```python
from build123d import *
from build123d.topology import SkipClean

# Parameters (mm, degrees)
SKETCH1_R                    = 4
COUPLER_SECTION_DEPTH        = 12.5
SKETCH3_R                    = 5
BEARING_SECTION_DEPTH        = 12
SKETCH4_R                    = 7
BEARING_STOP_DEPTH           = 3
SKETCH5_R                    = 4
SMALL_SEAL_SECTION_DEPTH     = 12.3
SET_SCREW_FLAT_SECTION_DEPTH = 10.5
SKETCH7_R                    = 4
IMPELLER_SECTION_DEPTH       = 22.163925
SKETCH8_R                    = 1.5
CUT_EXTRUDE1_DEPTH           = 8
CUT_EXTRUDE2_DEPTH           = 23
CUT_EXTRUDE2_DEPTH_BACK      = 23
SKETCH9_R                    = 1


with BuildPart() as part:
    # Sketch1 → coupler section (new body)
    with BuildSketch(Plane(origin=(0, 0, 0), x_dir=(1, 0, 0), z_dir=(0, 1, 0))):
        with Locations(Location((0, 0, 0), (0, 0, 270))):
            Circle(SKETCH1_R)
    extrude(amount=COUPLER_SECTION_DEPTH)

    # Sketch3 → bearing section (add)
    with BuildSketch(Plane(origin=(0, 12.5, 0), x_dir=(1, 0, 0), z_dir=(0, 1, 0))):
        with Locations(Location((0, 0, 0), (0, 0, 270))):
            Circle(SKETCH3_R)
    extrude(amount=BEARING_SECTION_DEPTH)

    # Sketch4 → bearing stop (add)
    with BuildSketch(Plane(origin=(0, 24.5, 0), x_dir=(1, 0, 0), z_dir=(0, 1, 0))):
        with Locations(Location((0, 0, 0), (0, 0, 270))):
            Circle(SKETCH4_R)
    extrude(amount=BEARING_STOP_DEPTH)

    # Sketch5 → small seal section (add)
    with BuildSketch(Plane(origin=(0, 27.5, 0), x_dir=(1, 0, 0), z_dir=(0, 1, 0))):
        with Locations(Location((0, 0, 0), (0, 0, 270))):
            Circle(SKETCH5_R)
    extrude(amount=SMALL_SEAL_SECTION_DEPTH)

    # Sketch6 → set screw flat section (cut)
    with BuildSketch(Plane.XZ):
        with BuildLine():
            Line((-2.645751311, 3), (2.645751311, 3))
            ThreePointArc((2.645751311, 3), (0, 4), (-2.645751311, 3))
        make_face()
    extrude(amount=-SET_SCREW_FLAT_SECTION_DEPTH, mode=Mode.SUBTRACT)

    # Sketch7 → impeller section (add)
    with BuildSketch(Plane(origin=(0, 39.8, 0), x_dir=(1, 0, 0), z_dir=(0, 1, 0))):
        with Locations(Location((0, 0, 0), (0, 0, 311.409622109))):
            Circle(SKETCH7_R)
    extrude(amount=IMPELLER_SECTION_DEPTH)

    # Sketch8 → Cut-Extrude1 (cut)
    with BuildSketch(Plane(origin=(0, 61.963925, 0), x_dir=(1, 0, 0), z_dir=(0, 1, 0))):
        with Locations(Location((0, 0, 0), (0, 0, 270))):
            Circle(SKETCH8_R)
    extrude(amount=-CUT_EXTRUDE1_DEPTH, mode=Mode.SUBTRACT)

    # Sketch9 → Cut-Extrude2 (cut, two sides: drawn at the far end of the back side and taken through both)
    with SkipClean():  # the faces are left unmerged after this step: merging them gives an invalid solid
        with BuildSketch(Plane.XY.offset(-CUT_EXTRUDE2_DEPTH_BACK)):
            with Locations(Location((0, 42.963925, 0), (0, 0, 89.999999996))):
                Circle(SKETCH9_R)
        extrude(amount=CUT_EXTRUDE2_DEPTH + CUT_EXTRUDE2_DEPTH_BACK, mode=Mode.SUBTRACT)


solid = part.part
```
Could you check a few things on this model? Use its own coordinates, in mm. A direction names the side the tool comes from. Coordinates: 2 decimals unless noted, no trailing zeros. Write each loop counter-clockwise with the first axis right and the second up, starting at its lowest first coordinate (ties: lowest second). Pieces come first, ordered by that corner, then holes. Notation, with made-up numbers: (14.25, 78) -> (70.25, 78) arc R18 ccw to (70.25, 86) -> close; hole circle Ø4 at (1.5, 56). An arc over 180 degrees is marked (long way). One line per question, with ' | ' between items. Start each with the question number.
1. Thinking about a two-plate mould opening in X: for faces 5 (the face through (-4.88, 18.42, -1.08)), 6 (the face through (-3, 27.5, 3)), 7 (the face through (0, 53.964, 0)), which applies, pulls with the +X half, pulls with the -X half, needs draft (parallel to the pull), parting line crosses it, or undercut?
2. For faces 1 (the face through (0, 6, -4)), 2 (the face through (1.2, 61.964, 1.3)), 3 (the face through (0, 5, 3)), 4 (the face through (0.45, 58.02, 1.43)), which set-ups out of +Z, -Z, +X, -X, +Y, -Y let a thin tool reach every point of the face, with its end or its side?
3. If we section it at B-B (y = 19): Please give me the cut outline in (x, z), and give its area (3 significant figures).
4. If we section it at D-D (y = 26): Please give me the cut outline in (x, z).
5. If we section it at A-A (z = -0.75): Please give me the cut outline in (x, y).
6. If we section it at C-C (x = 6.25): Please give me the cut outline in (y, z).
7. Will these pins go through, and if not, where does the flat tip stop? P1, Ø1, axis at x = 5, z = -1, coming from the -Y side; P2, Ø4, axis at y = 47, z = -1.5, coming from the -X side; P3, Ø4, axis at x = -0.5, z = -1, coming from the -Y side; P4, Ø0.8, axis at x = 0, z = 3.5, coming from the -Y side.
8. Please list where these lines run through material, in increasing order: line 1 along X through (y, z) = (59.5, 0); line 2 along Y through (x, z) = (4.5, -2.75); line 3 along Y through (x, z) = (3, 3.25).
Return value:
1) face 5: parting line crosses it | face 6: needs draft | face 7: undercut
2) face 1: -Y | face 2: +Z, -Z, +X, -X, +Y | face 3: +Z, +X, -X, -Y | face 4: +Y
3) outline: circle Ø10 at (0, 0) | area: 78.5 mm²
4) outline: circle Ø14 at (0, 0)
5) outline: (-6.96, 24.5) -> (-4.94, 24.5) -> (-4.94, 12.5) -> (-3.93, 12.5) -> (-3.93, 0) -> (3.93, 0) -> (3.93, 12.5) -> (4.94, 12.5) -> (4.94, 24.5) -> (6.96, 24.5) -> (6.96, 27.5) -> (3.93, 27.5) -> (3.93, 61.96) -> (1.3, 61.96) -> (1.3, 53.96) -> (-1.3, 53.96) -> (-1.3, 61.96) -> (-3.93, 61.96) -> (-3.93, 27.5) -> (-6.96, 27.5) -> close; hole circle Ø2 at (0, 42.96)
6) outline: (24.5, -3.15) -> (27.5, -3.15) -> (27.5, 3.15) -> (24.5, 3.15) -> close
7) P1: stops at y = 12.5 | P2: stops at x = -4 | P3: stops at y = 0 | P4: stops at y = 10.5
8) line 1: x = -4 to -1.5, 1.5 to 4 | line 2: y = 24.5 to 27.5 | line 3: y = 12.5 to 27.5
